Study the drawing (mm; zero at the part's minimum x, y, z) and answer. A direction names the side the tool comes from. Coordinates: 2 decimals unless noted, no trailing zeros. Order: outer loops, then holes, each group sorted by start corner. A loop starts at its lowest first (then second) coordinate and runs counter-clockwise, first axis right, second up. Notation, with made-up numbers: (11.25, 4) -> (26.25, 4) arc R7 ccw to (26.25, 16) -> close; hole circle Ø11 at (53, 30). An arc over 180 degrees is marked (long way). Write each question's results on one line, items separated by ' | '. Start each with the question number.
(1) The part is cut by section C-C, the plane x = 56.5. Give the vertices of the cut face in (y, z), then the cut area to 3 significant figures.
(2) The part is cut by section D-D, the plane y = 45. Give the vertices of the cut face in (x, z).
(3) Given pin 1 (18 mm diameter, centred on x = 60, z = 40, fed in from +Y); pin 2 (1 mm diameter, centred on y = 63, z = 11.5, fed in from -X); pin 3 (24 mm diameter, centred on x = 52.5, z = 20, fed in from +Y), each flat-ended and moving along its own axis, determine where each tip first touches the part or whether it passes through.
(4) Straight lines are drawn through the part: L1, parallel to X at y = 10, z = 40; L2, parallel to Y at x = 12.5, z = 40; L3, parallel to X at y = 91.5, z = 30. For each, find the intervals that lie inside material, in ascending order.
(5) The part is cut by section B-B, the plane y = 58.5. Give the vertices of the cut face in (x, z).
(6) Determine the mould class of the marked faces 5, 6, 7 and 8 for opening direction Z: +Z half, -Z half, draft (parallel to the pull), parting line (faces both ways), or undercut.
(7) A tool of negligible diameter and unlimited length cuts with its end or side. For the marked faces 1, 2, 3 and 4, from which of +Z, -Z, +X, -X, +Y, -Y can it reach the whole face along a straight path? Write none if from no direction.
(8) The part is cut by section A-A, the plane z = 40. Give the vertices of the cut face in (x, y), then the cut area to 3 significant figures.
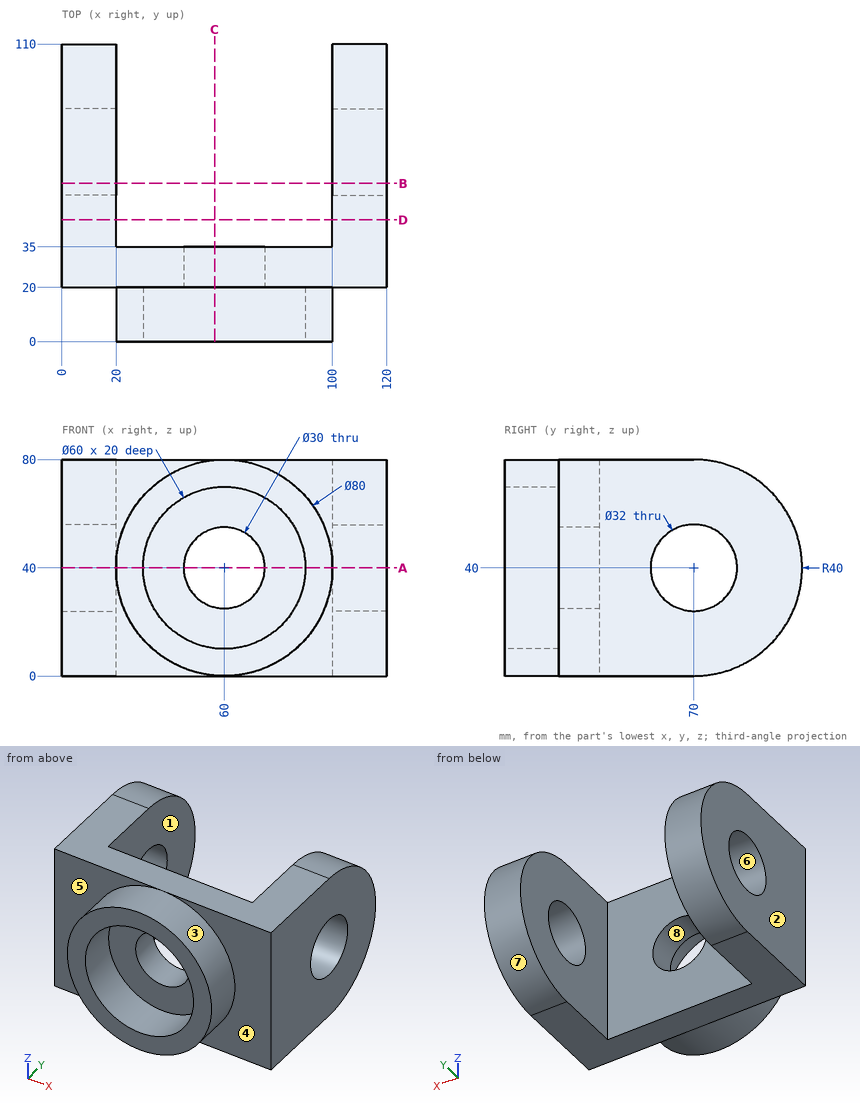
Established:
1) outline: (0, 0.15) -> (20, 0.15) -> (20, 0) -> (35, 0) -> (35, 25.41) -> (20, 25.41) -> (20, 10.2) -> (0, 10.2) -> close; (0, 69.8) -> (20, 69.8) -> (20, 54.59) -> (35, 54.59) -> (35, 80) -> (20, 80) -> (20, 79.85) -> (0, 79.85) -> close | area: 1,160 mm^2
2) outline: (0, 0) -> (20, 0) -> (20, 80) -> (0, 80) -> close; (100, 0) -> (120, 0) -> (120, 80) -> (100, 80) -> close
3) pin 1: passes through | pin 2: stops at x = 0 | pin 3: stops at y = 35
4) L1: x = 20 to 30, 90 to 100 | L2: y = 20 to 54, 86 to 110 | L3: x = 0 to 20, 100 to 120
5) outline: (0, 0) -> (20, 0) -> (20, 28.88) -> (0, 28.88) -> close; (0, 51.12) -> (20, 51.12) -> (20, 80) -> (0, 80) -> close; (100, 0) -> (120, 0) -> (120, 28.88) -> (100, 28.88) -> close; (100, 51.12) -> (120, 51.12) -> (120, 80) -> (100, 80) -> close
6) face 5: draft | face 6: undercut | face 7: parting line | face 8: undercut
7) face 1: +Z, -Z, +Y | face 2: +Z, -Z, -X, +Y, -Y | face 3: -Y | face 4: +X, -Y
8) outline: (0, 20) -> (20, 20) -> (20, 0) -> (30, 0) -> (30, 20) -> (45, 20) -> (45, 35) -> (20, 35) -> (20, 54) -> (0, 54) -> close; (0, 86) -> (20, 86) -> (20, 110) -> (0, 110) -> close; (75, 20) -> (90, 20) -> (90, 0) -> (100, 0) -> (100, 20) -> (120, 20) -> (120, 54) -> (100, 54) -> (100, 35) -> (75, 35) -> close; (100, 86) -> (120, 86) -> (120, 110) -> (100, 110) -> close | area: 3,470 mm^2
